Autodesk Inventor part; units mm, degrees
ref_plane "YZ Plane" through (0, 0, 0) normal (1, 0, 0) x (0, 1, 0)
ref_plane "XZ Plane" through (0, 0, 0) normal (0, 1, 0) x (-1, 0, 0)
ref_plane "XY Plane" through (0, 0, 0) normal (0, 0, 1) x (1, 0, 0)
sketch "Sketch2" plane through (0, 0, 0) normal (1, 0, 0) x (0, 1, 0)
  line L0 (0.8, -9.1) -> (-0.8, -9.1)
  line L1 (0.8, -9.1) -> (0.8, -1.4)
  line L2 (0, 1.82) -> (0, -10.92)
  line L3 (0, -9.1) -> (0.8, -9.1)
  line L4 (0.8, -6.902) -> (0, -9.1)
  point P0 (0, 0)
  dimension "d55" = 20
sketch "Sketch1" plane through (0, 0, 0) normal (1, 0, 0) x (0, 1, 0)
  line L0 (0, 0) -> (0, -197.906)
  line L1 (0, 0) -> (-1.6, 0)
  line L2 (-1.6, 0) -> (-1.6, -1.1)
  line L3 (-1.6, -1.1) -> (-0.8, -1.1)
  line L4 (-0.8, -1.1) -> (-0.8, -9.1)
  line L5 (0, -9.1) -> (-0.8, -9.1)
  dimension "d0" = 3.2
  dimension "d4" = 1.6
  dimension "d5" = 1.1
  dimension "d42" = 8
revolve "Revolution1" add sketch "Sketch1" angle 360 about axis through (0, 0, 0) along (0, 0, -1)
fillet "Fillet1" radius 0.3 1 edges at (0, 0.8, -1.1)
thread "Thread1"
revolve "Revolution2" cut sketch "Sketch2" angle 360 about axis through (0, 0, 0) along (0, 0, -1)
sketch "Sketch3" plane through (0, 0, 0) normal (1, 0, 0) x (0, 1, 0)
  line L0 (-0.2, 0) -> (0.2, 0)
  line L1 (0.2, 0) -> (0.2, -0.55)
  line L2 (0.2, -0.55) -> (-0.2, -0.55)
  line L3 (-0.2, -0.55) -> (-0.2, 0)
  point P0 (0, 0)
  point P1 (0, 0)
  dimension "d29" = 0.4
  dimension "d30" = 0.55
extrude "Extrusion1" cut sketch "Sketch3" along normal through all both and the other way through all
sketch "Sketch4" plane through (0, 0, 0) normal (1, 0, 0) x (0, 1, 0)
  line L0 (0.2, 0) -> (0.2, 0)
  arc A0 (1.6, -0.5506) -> (0, 0) centre (0, -2.6) ccw
  line L1 (1.6, 0) -> (0.2, 0)
  line L2 (1.6, -1.1) -> (1.6, 0)
  line L3 (0.2, 0) -> (0, 0)
  line L4 (0, -3.1468) -> (0, 0.6806)
  dimension "d40" = 2.6
revolve "Revolution3" cut sketch "Sketch4" angle 360 about axis through (0, 0, -10) along (0, 0, 1)
equation "\"d44\" = r"
equation "\"d45\" = GEL"
equation "\"d29\" = SBR"
equation "\"d30\" = STI"
equation "\"d40\" = R1"
equation "\"d0\" = KOD"
equation "\"d4\" = NND"
equation "\"d5\" = KOH"
equation "\"d42\" = NLG"
equation "\"KOD\" = 3.2"
equation "\"NND\" = 1.6"
equation "\"NLG\" = 8"
equation "\"KOH\" = 1.1"
equation "\"R1\" = 2.6"
equation "\"r\" = 0.3"
equation "\"SBR\" = 0.4"
equation "\"STI\" = 0.55"
equation "\"GEL\" = 0.6 * NLG"
properties part number "DIN 96 - 1,6x8" material "Stahl"
CAD build for the part. Positions are in the model's coordinates, mm. A direction names the side the tool comes from. Coordinates: 2 decimals unless noted, no trailing zeros. Write each loop counter-clockwise with the first axis right and the second up, starting at its lowest first coordinate (ties: lowest second). Pieces come first, ordered by that corner, then holes. Notation, with made-up numbers: (67.25, 71.25) -> (111.25, 71.25) arc R36 ccw to (111.25, 105.25) -> close; hole circle Ø11 at (2, 30). An arc over 180 degrees is marked (long way). Use CSV: the item, a comma, the result in double quotes. Start each with the question number.
Item 1: Tool access for faces 1 (the cylindrical face through (0.49, 0.63, -4.19)), 2 (the cylindrical face through (0.97, 1.27, -0.83)): list every direction of +Z, -Z, +X, -X, +Y, -Y with a clear straight run to the whole face (end or side of a thin tool).
Item 2: Band-saw the part on B-B, the plane z = -1. Write the cut outline in (x, y), plus the area to 3 significant figures.
Item 3: Wall check: probe 1 along X at (y, z) = (0.05, -2.75); probe 2 along Y at (x, z) = (0.7, -2.25). Give the ranges that are in metal, low to high.
Item 4: Band-saw the part on A-A, the plane z = -5.75. Write the cut outline in (x, y), plus the area to 3 significant figures.
Response values:
1,face 1,"-Z"
1,face 2,"+Z, -Z"
2,outline,"circle Ø3.2 at (0, 0)"
2,area,"8.04 mm2"
3,probe 1,"x = -0.8 to 0.8"
3,probe 2,"y = -0.39 to 0.39"
4,outline,"circle Ø1.6 at (0, 0)"
4,area,"2.01 mm2"
